```python
from build123d import *

# Parameters (mm, degrees)
F0_R     = 2.45
F1_DEPTH = 460


# Not quite as in the source:
# - ends of sketch curves that miss each other by under 0.0002 mm in the source are joined


with BuildPart() as f1:
    # F0 (on Front) → F1 (new body)
    with BuildSketch(Plane.XZ):
        with BuildLine():
            Line((-3.1749674082, 15), (-12, 15))
            ThreePointArc((-12, 15), (-14.1213203436, 14.1213203436), (-15, 12))
            Line((-15, 12), (-15, 3.175))
            Line((-15, 3.175), (-13.0855346263, 3.175))
            ThreePointArc((-13.0855346263, 3.175), (-12.3835980145, 3.4627605788), (-12.0856407741, 4.1604300138))
            Line((-12.0856407741, 4.1604300138), (-12.0761692778, 4.8104300138))
            ThreePointArc((-12.0761692778, 4.8104300138), (-12.3638237087, 5.5269366118), (-13.0760631299, 5.825))
            Line((-13.0760631299, 5.825), (-13.5, 5.825))
            Line((-13.5, 5.825), (-13.5, 8.225))
            Line((-13.5, 8.225), (-9.8968845016, 8.225))
            ThreePointArc((-9.8968845016, 8.225), (-9.5279915195, 8.1544718757), (-9.2111331975, 7.9528359354))
            Line((-9.2111331975, 7.9528359354), (-5.4142486959, 4.3754933338))
            ThreePointArc((-5.4142486959, 4.3754933338), (-5.1819174045, 4.0440465354), (-5.1, 3.6476573984))
            Line((-5.1, 3.6476573984), (-5.1, -3.4999243287))
            ThreePointArc((-5.1, -3.4999243287), (-5.1782354607, -3.8876744211), (-5.4007002683, -4.2147528992))
            Line((-5.4007002683, -4.2147528992), (-9.2084959767, -7.9398285705))
            ThreePointArc((-9.2084959767, -7.9398285705), (-9.5301904718, -8.1509666761), (-9.9077957084, -8.225))
            Line((-9.9077957084, -8.225), (-13.5, -8.225))
            Line((-13.5, -8.225), (-13.5, -5.825))
            Line((-13.5, -5.825), (-13.0760631299, -5.825))
            ThreePointArc((-13.0760631299, -5.825), (-12.3638237087, -5.5269366118), (-12.0761692778, -4.8104300138))
            Line((-12.0761692778, -4.8104300138), (-12.0856407741, -4.1604300138))
            ThreePointArc((-12.0856407741, -4.1604300138), (-12.3835980145, -3.4627605788), (-13.0855346263, -3.175))
            Line((-13.0855346263, -3.175), (-15, -3.175))
            Line((-15, -3.175), (-15, -12))
            ThreePointArc((-15, -12), (-14.1213203436, -14.1213203436), (-12, -15))
            Line((-12, -15), (-3.175, -15))
            Line((-3.175, -15), (-3.175, -13.0855346263))
            ThreePointArc((-3.175, -13.0855346263), (-3.4627605788, -12.3835980145), (-4.1604300138, -12.0856407741))
            Line((-4.1604300138, -12.0856407741), (-4.8104300138, -12.0761692778))
            ThreePointArc((-4.8104300138, -12.0761692778), (-5.5269366118, -12.3638237087), (-5.825, -13.0760631299))
            Line((-5.825, -13.0760631299), (-5.825, -13.5))
            Line((-5.825, -13.5), (-8.225, -13.5))
            Line((-8.225, -13.5), (-8.225, -9.8968845016))
            ThreePointArc((-8.225, -9.8968845016), (-8.1544718757, -9.5279915195), (-7.9528359354, -9.2111331975))
            Line((-7.9528359354, -9.2111331975), (-4.3754933338, -5.4142486959))
            ThreePointArc((-4.3754933338, -5.4142486959), (-4.0440465354, -5.1819174045), (-3.6476573984, -5.1))
            Line((-3.6476573984, -5.1), (3.4999243287, -5.1))
            ThreePointArc((3.4999243287, -5.1), (3.8876744211, -5.1782354607), (4.2147528992, -5.4007002683))
            Line((4.2147528992, -5.4007002683), (7.9398285705, -9.2084959767))
            ThreePointArc((7.9398285705, -9.2084959767), (8.1509666761, -9.5301904718), (8.225, -9.9077957084))
            Line((8.225, -9.9077957084), (8.225, -13.5))
            Line((8.225, -13.5), (5.825, -13.5))
            Line((5.825, -13.5), (5.825, -13.0760631299))
            ThreePointArc((5.825, -13.0760631299), (5.5269366118, -12.3638237087), (4.8104300138, -12.0761692778))
            Line((4.8104300138, -12.0761692778), (4.1604300138, -12.0856407741))
            ThreePointArc((4.1604300138, -12.0856407741), (3.4627605788, -12.3835980145), (3.175, -13.0855346263))
            Line((3.175, -13.0855346263), (3.175, -15))
            Line((3.175, -15), (12, -15))
            ThreePointArc((12, -15), (14.1213203436, -14.1213203436), (15, -12))
            Line((15, -12), (15, -3.175))
            Line((15, -3.175), (13.0855346263, -3.175))
            ThreePointArc((13.0855346263, -3.175), (12.3835980145, -3.4627605788), (12.0856407741, -4.1604300138))
            Line((12.0856407741, -4.1604300138), (12.0761692778, -4.8104300138))
            ThreePointArc((12.0761692778, -4.8104300138), (12.3638237087, -5.5269366118), (13.0760631299, -5.825))
            Line((13.0760631299, -5.825), (13.5, -5.825))
            Line((13.5, -5.825), (13.5, -8.225))
            Line((13.5, -8.225), (9.9077957084, -8.225))
            ThreePointArc((9.9077957084, -8.225), (9.5301904718, -8.1509666761), (9.2084959767, -7.9398285705))
            Line((9.2084959767, -7.9398285705), (5.4007002683, -4.2147528992))
            ThreePointArc((5.4007002683, -4.2147528992), (5.1782354607, -3.8876744211), (5.1, -3.4999243287))
            Line((5.1, -3.4999243287), (5.1, 3.6476573984))
            ThreePointArc((5.1, 3.6476573984), (5.1819174045, 4.0440465354), (5.4142486959, 4.3754933338))
            Line((5.4142486959, 4.3754933338), (9.2111331975, 7.9528359354))
            ThreePointArc((9.2111331975, 7.9528359354), (9.5279915195, 8.1544718757), (9.8968845016, 8.225))
            Line((9.8968845016, 8.225), (13.5, 8.225))
            Line((13.5, 8.225), (13.5, 5.825))
            Line((13.5, 5.825), (13.0760631299, 5.825))
            ThreePointArc((13.0760631299, 5.825), (12.3638237087, 5.5269366118), (12.0761692778, 4.8104300138))
            Line((12.0761692778, 4.8104300138), (12.0856407741, 4.1604300138))
            ThreePointArc((12.0856407741, 4.1604300138), (12.3835980145, 3.4627605788), (13.0855346263, 3.175))
            Line((13.0855346263, 3.175), (15, 3.175))
            Line((15, 3.175), (15, 12))
            ThreePointArc((15, 12), (14.1213203436, 14.1213203436), (12, 15))
            Line((12, 15), (3.1750325918, 15))
            Line((3.1750325918, 15), (3.1750325918, 13.0854824722))
            ThreePointArc((3.1750325918, 13.0854824722), (3.4627931706, 12.3835458604), (4.1604626057, 12.0855886201))
            Line((4.1604626057, 12.0855886201), (4.8104626057, 12.0761171237))
            ThreePointArc((4.8104626057, 12.0761171237), (5.5269692036, 12.3637715546), (5.8250325918, 13.0760109758))
            Line((5.8250325918, 13.0760109758), (5.8250325918, 13.4999478459))
            Line((5.8250325918, 13.4999478459), (8.2250325918, 13.4999478459))
            Line((8.2250325918, 13.4999478459), (8.2250325918, 9.8968323476))
            ThreePointArc((8.2250325918, 9.8968323476), (8.1545044675, 9.5279393654), (7.9528685272, 9.2110810434))
            Line((7.9528685272, 9.2110810434), (4.3755259256, 5.4141965418))
            ThreePointArc((4.3755259256, 5.4141965418), (4.0440791272, 5.1818652505), (3.6476899902, 5.0999478459))
            Line((3.6476899902, 5.0999478459), (-3.4998917369, 5.0999478459))
            ThreePointArc((-3.4998917369, 5.0999478459), (-3.8876418293, 5.1781833067), (-4.2147203074, 5.4006481142))
            Line((-4.2147203074, 5.4006481142), (-7.9397959787, 9.2084438226))
            ThreePointArc((-7.9397959787, 9.2084438226), (-8.1509340843, 9.5301383177), (-8.2249674082, 9.9077435543))
            Line((-8.2249674082, 9.9077435543), (-8.2249674082, 13.4999478459))
            Line((-8.2249674082, 13.4999478459), (-5.8249674082, 13.4999478459))
            Line((-5.8249674082, 13.4999478459), (-5.8249674082, 13.0760109758))
            ThreePointArc((-5.8249674082, 13.0760109758), (-5.5269040199, 12.3637715546), (-4.810397422, 12.0761171237))
            Line((-4.810397422, 12.0761171237), (-4.160397422, 12.0855886201))
            ThreePointArc((-4.160397422, 12.0855886201), (-3.462727987, 12.3835458604), (-3.1749674082, 13.0854824722))
            Line((-3.1749674082, 13.0854824722), (-3.1749674082, 15))
        make_face()
        with BuildLine():
            Line((-13.5, -11.5), (-13.5, -9.7))
            Line((-13.5, -9.7), (-9.7, -9.7))
            Line((-9.7, -9.7), (-9.7, -13.5))
            Line((-9.7, -13.5), (-11.5, -13.5))
            ThreePointArc((-11.5, -13.5), (-12.9142135624, -12.9142135624), (-13.5, -11.5))
        make_face(mode=Mode.SUBTRACT)
        with BuildLine():
            Line((9.7, -9.7), (13.5, -9.7))
            Line((13.5, -9.7), (13.5, -11.5))
            ThreePointArc((13.5, -11.5), (12.9142135624, -12.9142135624), (11.5, -13.5))
            Line((11.5, -13.5), (9.7, -13.5))
            Line((9.7, -13.5), (9.7, -9.7))
        make_face(mode=Mode.SUBTRACT)
        with BuildLine():
            ThreePointArc((-13.5, 11.5), (-12.9142135624, 12.9142135624), (-11.5, 13.5))
            Line((-11.5, 13.5), (-9.7, 13.5))
            Line((-9.7, 13.5), (-9.7, 9.7))
            Line((-9.7, 9.7), (-13.5, 9.7))
            Line((-13.5, 9.7), (-13.5, 11.5))
        make_face(mode=Mode.SUBTRACT)
        Circle(F0_R, mode=Mode.SUBTRACT)
        with BuildLine():
            Line((9.7, 13.5), (11.5, 13.5))
            ThreePointArc((11.5, 13.5), (12.9142135624, 12.9142135624), (13.5, 11.5))
            Line((13.5, 11.5), (13.5, 9.7))
            Line((13.5, 9.7), (9.7, 9.7))
            Line((9.7, 9.7), (9.7, 13.5))
        make_face(mode=Mode.SUBTRACT)
    extrude(amount=F1_DEPTH)


solid = f1.part
```
Input: part model. Units: mm. Frame: model coordinates. Round coordinates to 2 decimals unless told otherwise and drop trailing zeros. Write each question's results on one line, items separated by ' | '.
Q1. Draft query along X for faces 1 (the face through (8, -227, 15)), 2 (the face through (0, -227, 5.1)), 3 (the face through (15, -227, -8)). Return one class per face: released by +X, released by -X, zero draft, split by the parting line, or undercut.
Results:
face 1: zero draft | face 2: undercut | face 3: released by +X
Q2. Pin query (flat end, axial travel): P1, Ø0.5, axis at y = -302, z = 13.5, coming from the +X side; P2, Ø2, axis at y = -281.5, z = 14, coming from the -X side; P3, Ø2, axis at y = -221, z = 14.5, coming from the +X side. Return the tip coordinate at first contact, or that it passes through.
Results:
P1: stops at x = 14.73 | P2: stops at x = -14.83 | P3: stops at x = 14.6
Q3. Section query A-A (y = -329). State how many separate pieces and enclosed holes the cut face has, and give its area (3 significant figures).
Results:
separate pieces: 1 | enclosed holes: 5 | area: 330 mm^2
Q4. Line query: line 1 along Z through (x, y) = (-10, -433.5) (3 decimals); line 2 along Z through (x, y) = (-12, -209) (1 decimal); line 3 along X through (y, z) = (-163, -5.5). Output: solid intervals per line, ascending.
Results:
line 1: z = -15 to -13.5, -9.7 to -8.225, 8.225 to 9.7, 13.5 to 15 | line 2: z = -15 to -13.4, -9.7 to -8.2, 8.2 to 9.7, 13.4 to 15 | line 3: x = -15 to -12.34, -6.71 to -4.46, 4.31 to 6.71, 12.34 to 15
